Here's how the part is built. I have some questions about the finished solid (model axes, mm). Round coordinates to 2 decimals unless told otherwise and drop trailing zeros. Loops run counter-clockwise (first coordinate to the right, second up) from the corner with the lowest first, then second, coordinate; pieces in that order, holes last. Notation, with made-up numbers: M -23.5,88.25 L 30.5,88.25 A23 cw 30.5,121.25 Z; hole C 52,51.25 d1. An arc over 180 degrees is marked long. Use a Markdown table: item, result.
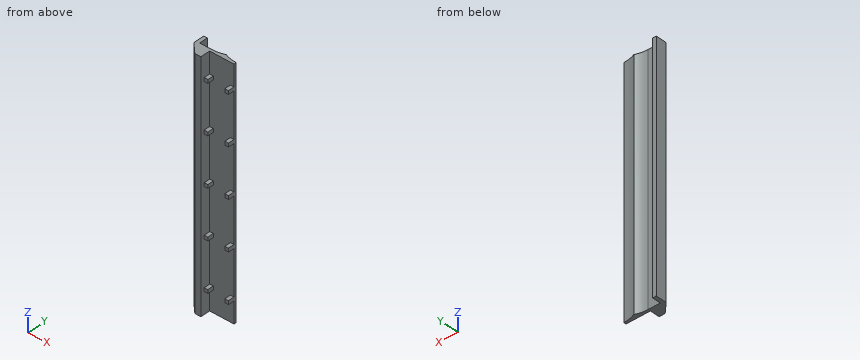
Autodesk Inventor part; units mm, degrees
ref_plane "YZ Plane" through (0, 0, 0) normal (1, 0, 0) x (0, 1, 0)
ref_plane "XZ Plane" through (0, 0, 0) normal (0, 1, 0) x (-1, 0, 0)
ref_plane "XY Plane" through (0, 0, 0) normal (0, 0, 1) x (1, 0, 0)
sketch "スケッチ1" plane through (0, 0, 0) normal (0, 1, 0) x (-1, 0, 0)
  line L0 (0, 99) -> (20, 99)
  line L1 (20, 99) -> (20, -99)
  line L2 (20, -99) -> (0, -99)
  line L3 (0, -99) -> (0, 99)
  line L4 (20, -99) -> (20, -109)
  line L5 (20, -109) -> (9, -109)
  line L6 (9, -109) -> (11, -99)
  line L7 (10.5, 99) -> (8.5, 88.5)
  line L8 (8.5, 88.5) -> (20, 88.5)
  point P0 (0, 0)
  point P1 (0, 0)
  point P2 (10, -99)
  point P3 (10, 99)
  dimension "d0" = 198
  dimension "d1" = 20
  dimension "d4" = 10
  dimension "d5" = 1
  dimension "d6" = 1
  dimension "d7" = 10.5
  dimension "d8" = 1.5
  dimension "d9" = 0.5
extrude "押し出し1" add sketch "スケッチ1" along normal blind 5.5 contours L0 L7 L8 L1 L2 L3 | L2 L4 L5 L6
sketch "スケッチ2" plane through (0, 5.5, 0) normal (0, 1, 0) x (1, 0, 0)
  line L0 (-20, 109) -> (-20, -88.5)
  line L1 (-20, -1.5) -> (-17, -1.5)
  line L2 (-17, -1.5) -> (-17, 1.5)
  line L3 (-17, 1.5) -> (-20, 1.5)
  line L4 (-20, 1.5) -> (-20, -1.5)
  line L5 (0, -99) -> (0, 99)
  line L6 (0, -1.5) -> (-3, -1.5)
  line L7 (-3, -1.5) -> (-3, 1.5)
  line L8 (-3, 1.5) -> (0, 1.5)
  line L9 (0, 1.5) -> (0, -1.5)
  point P0 (0, 0)
  point P1 (-17, 0)
  point P2 (0, 0)
  point P3 (0, 1.5)
  dimension "d10" = 3
  dimension "d11" = 3
extrude "押し出し2" cut sketch "スケッチ2" against normal through all
pattern_linear "矩形状パターン1" count 3 spacing 40 along (0, 0, -1) count 3 spacing 40 along (0, 0, 1) of "押し出し2"
sketch "スケッチ3" plane through (0, 5.5, 0) normal (0, 1, 0) x (1, 0, 0)
  line L0 (-20, -88.5) -> (-8.5, -88.5)
  line L1 (-20, -99) -> (0, -99)
  line L2 (0, -99) -> (0, 99)
  line L3 (-20, 109) -> (-20, -88.4991)
  line L4 (-20, -38.5) -> (-17, -38.5)
  line L5 (-17, -38.5) -> (-17, -41.5)
  line L6 (-17, -41.5) -> (-20, -41.5)
  line L7 (-20, -41.5) -> (-20, -78.5)
  line L8 (-20, -78.5) -> (-17, -78.5)
  line L9 (-17, -78.5) -> (-17, -81.5)
  line L10 (-17, -81.5) -> (-20, -81.5)
  line L11 (-20, -81.5) -> (-20, -88.5)
  line L12 (-20, -88.5) -> (-8.5, -88.5)
  line L13 (-8.5, -88.5) -> (-10.5, -99)
  line L14 (-10.5, -99) -> (0, -99)
  line L15 (0, -99) -> (0, -81.5)
  line L16 (0, -81.5) -> (-3, -81.5)
  line L17 (-3, -81.5) -> (-3, -78.5)
  line L18 (-3, -78.5) -> (0, -78.5)
  line L19 (0, -78.5) -> (0, -41.5)
  line L20 (0, -41.5) -> (-3, -41.5)
  line L21 (-3, -41.5) -> (-3, -38.5)
  line L22 (-3, -38.5) -> (0, -38.5)
  line L23 (0, -38.5) -> (0, -1.5)
  line L24 (0, -1.5) -> (-3, -1.5)
  line L25 (-3, -1.5) -> (-3, 1.5)
  line L26 (-3, 1.5) -> (0, 1.5)
  line L27 (0, 1.5) -> (0, 38.5)
  line L28 (0, 38.5) -> (-3, 38.5)
  line L29 (-3, 38.5) -> (-3, 41.5)
  line L30 (-3, 41.5) -> (0, 41.5)
  line L31 (0, 41.5) -> (0, 78.5)
  line L32 (0, 78.5) -> (-3, 78.5)
  line L33 (-3, 78.5) -> (-3, 81.5)
  line L34 (-3, 81.5) -> (0, 81.5)
  line L35 (0, 81.5) -> (0, 99)
  line L36 (-9, 109) -> (-20, 109)
  line L37 (-20, 109) -> (-20, 81.5)
  line L38 (-20, 81.5) -> (-17, 81.5)
  line L39 (-17, 81.5) -> (-17, 78.5)
  line L40 (-17, 78.5) -> (-20, 78.5)
  line L41 (-20, 78.5) -> (-20, 41.5)
  line L42 (-20, 41.5) -> (-17, 41.5)
  line L43 (-17, 41.5) -> (-17, 38.5)
  line L44 (-17, 38.5) -> (-20, 38.5)
  line L45 (-20, 38.5) -> (-20, 1.5)
  line L46 (-20, 1.5) -> (-17, 1.5)
  line L47 (-17, 1.5) -> (-17, -1.5)
  line L48 (-17, -1.5) -> (-20, -1.5)
  line L49 (-20, -1.5) -> (-20, -38.5)
  line L50 (-20, 109) -> (-20, 81.5)
  line L51 (-20, -99) -> (-20, -88.4991)
  line L52 (-9, 109) -> (0, 109)
  line L53 (0, 99) -> (0, 109)
  line L54 (0, 99) -> (-20, 99)
  point P0 (0, 0)
  point P1 (-11, 99)
  point P2 (0, -78.5)
  point P3 (0, -38.5)
  point P4 (0, 41.5)
  point P5 (0, 81.5)
  point P6 (-20, -88.4991)
extrude "押し出し3" cut sketch "スケッチ3" against normal through all contours L3 L10 L9 L8 L6 L5 L4 L48 L47 L46 L44 L43 L42 L40 L39 L38 L54 L2 L34 L33 L32 L30 L29 L28 L26 L25 L24 L22 L21 L20 L18 L17 L16 L1 L13 L0 | L3 L8 L9 L10 | L3 L4 L5 L6 | L16 L17 L18 L2 | L3 L46 L47 L48 | L20 L21 L22 L2 | L3 L42 L43 L44 | L24 L25 L26 L2 | L3 L38 L39 L40 | L28 L29 L30 L2 | L3 L36 L52 L53 L54 | L32 L33 L34 L2
extrude "押し出し4" add sketch "スケッチ3" against normal blind 5 contours L3 L8 L9 L10 | L3 L4 L5 L6 | L16 L17 L18 L2 | L3 L46 L47 L48 | L20 L21 L22 L2 | L3 L42 L43 L44 | L24 L25 L26 L2 | L3 L38 L39 L40 | L28 L29 L30 L2 | L32 L33 L34 L2
extrude "押し出し5" add sketch "スケッチ3" along normal blind 2 contours L3 L10 L9 L8 L6 L5 L4 L48 L47 L46 L44 L43 L42 L40 L39 L38 L54 L2 L34 L33 L32 L30 L29 L28 L26 L25 L24 L22 L21 L20 L18 L17 L16 L1 L13 L0 | L0 L13 L1 L51 | L3 L8 L9 L10 | L3 L4 L5 L6 | L16 L17 L18 L2 | L3 L46 L47 L48 | L20 L21 L22 L2 | L3 L42 L43 L44 | L24 L25 L26 L2 | L3 L38 L39 L40 | L28 L29 L30 L2 | L32 L33 L34 L2
sketch "スケッチ4" plane through (-20, 5.5, 99) normal (0, 0, 1) x (1, 0, 0)
  arc A0 (0, 2) -> (10, 4) centre (0, 28) ccw
  line L0 (0, 2) -> (20, 2)
  arc A1 (10, 4) -> (20, 2) centre (20, 28) ccw
  line L1 (10, 4) -> (10, 2) construction
  point P0 (20, -5.5)
  point P1 (14.6904, 2)
  point P2 (5.3096, 2)
  dimension "d27" = 2
extrude "押し出し6" add sketch "スケッチ4" against normal up to surface (198 mm away)
sketch "スケッチ8" plane through (-20, 5.5, 99) normal (0, 0, 1) x (1, 0, 0)
  arc A0 (0, 2) -> (10, 4) centre (0, 28) ccw
  line L0 (0, 2) -> (-10, 2)
  line L1 (-10, 2) -> (-10, -8)
  line L2 (-10, -8) -> (0, -8)
  line L3 (0, -8) -> (0, 2)
  line L4 (-10, -8) -> (-13, -8)
  line L5 (-13, -8) -> (-13, 9)
  line L6 (-13, 9) -> (-10, 9)
  line L7 (-10, 9) -> (-10, -8)
  point P0 (20, -5.5)
  dimension "d44" = 7
  dimension "d45" = 3
  dimension "d46" = 10
  dimension "d47" = 10
extrude "押し出し9" add sketch "スケッチ8" against normal up to surface (198 mm away)
chamfer "面取り3" distance 8 angle 45 1 edges at (-33, -2.5, 0)
properties part number "front_rail"
Q1. Imagine slicing it at A-A, the plane z = -61.5. Please give me the cut outline in (x, y).
Return value:
| item | result |
|---|---|
| outline | M -33,5.5 L -25,-2.5 L -20,-2.5 L -20,5.5 L 0,5.5 L 0,7.5 A26 cw -10,9.5 A26 cw -20,7.5 L -30,7.5 L -30,14.5 L -33,14.5 Z |
Q2. Imagine slicing it at D-D, the plane y = 11.5. Please give me the cut outline in (x, z).
Return value:
| item | result |
|---|---|
| outline | M -33,-99 L -30,-99 L -30,99 L -33,99 Z |
Q3. I need wall thicknesses on line 1 (X direction, y = 12.75, z = -86); line 2 (Y direction, x = -29, z = 84.5); line 3 (Y direction, x = -27.5, z = -61). Which ranges of each line are inside material? Lowest first, please. Write a range as from..to.
Return value:
| item | result |
|---|---|
| line 1 | x = -33..-30 |
| line 2 | y = 1.5..7.5 |
| line 3 | y = 0..7.5 |
Q4. Imagine slicing it at B-B, the plane y = 2.75. Give the number of separate pieces and of enclosed holes in the cut face, then the cut area to 3 significant figures.
Return value:
| item | result |
|---|---|
| separate pieces | 6 |
| enclosed holes | 0 |
| area | 2,120 mm^2 |
Q5. Will these pins go through, and if not, where does the flat tip stop? P1, Ø1.5, axis at x = -18.5, y = 2.5, coming from the +Z side; P2, Ø1.5, axis at x = -1, z = 40, coming from the -Y side; P3, Ø0.9, axis at x = -18.5, y = 2, coming from the -Z side.
Return value:
| item | result |
|---|---|
| P1 | stops at z = 81.5 |
| P2 | stops at y = 0.5 |
| P3 | stops at z = -81.5 |
Q6. Imagine slicing it at C-C, the plane x = -27. Please give me the cut outline in (y, z), then the cut area to 3 significant figures.
Return value:
| item | result |
|---|---|
| outline | M -0.5,-99 L 7.5,-99 L 7.5,99 L -0.5,99 Z |
| area | 1,580 mm^2 |
